Work out the finished part from the listing and answer in its coordinate system (mm). A direction names the side the tool comes from. Coordinates: 2 decimals unless noted, no trailing zeros. Order: outer loops, then holes, each group sorted by start corner. A loop starts at its lowest first (then second) coordinate and runs counter-clockwise, first axis right, second up. Notation, with made-up numbers: (-13.5, 35) -> (25.5, 35) arc R32 cw to (25.5, 71) -> close; hole circle Ø6 at (84.5, -32.75). An arc over 180 degrees is marked (long way). Answer as CSV lines item,"result". Start each with the question number.
Item 1: Section C-C (y = 26) is taken. Write down the section's boundary in (x, z), then the cut area to 3 significant figures.
Item 2: Straight lines are drawn through the part: L1, parallel to Y at x = 417.5, z = -29.5; L2, parallel to Z at x = -344, y = 48. For each, find the intervals that lie inside material, in ascending order.
Item 3: Each of these flat-tipped pins is pushed along its axis until it touches: pin 1 Ø3 at (x, y) = (123, 39.5) entering from -Z; pin 2 Ø1 at (x, z) = (-215.5, -22.5) entering from +Y. Where does it stop, or does it pass through?
Item 4: Section A-A (x = 196) is taken. Write down the section's boundary in (y, z).
Item 5: Section B-B (z = -20) is taken. Write down the section's boundary in (x, y), then the cut area to 3 significant figures.
Item 6: Which of the six approach directions +Z, -Z, +X, -X, +Y, -Y give full straight-line access (tool end or side, diameter ignored) to faces 1 (the face through (8, 32, 0)), 2 (the face through (8, 32, -3))?
```python
from build123d import *

# Parameters (mm, degrees)
BOSS_EXTRUDE1_DEPTH = 550
FILLET1_R           = 5
FILLET2_R           = 1


with BuildPart() as part:
    # Sketch1 → Boss-Extrude1 (new, symmetric)
    with BuildSketch(Plane(origin=(0, 0, 0), x_dir=(0, 0, -1), z_dir=(1, 0, 0))):
        Polygon((0, 0), (0, 60), (3, 60), (3, 3), (60, 3), (60, 0), align=None)
    extrude(amount=BOSS_EXTRUDE1_DEPTH, both=True)

    # Fillet1
    fillet1_edges = [part.edges().sort_by_distance(p)[0] for p in [
        (0, 0, 0),
    ]]
    fillet(fillet1_edges, radius=FILLET1_R)

    # Fillet2
    fillet2_edges = [part.edges().sort_by_distance(p)[0] for p in [
        (0, 3, -3),
    ]]
    fillet(fillet2_edges, radius=FILLET2_R)


solid = part.part
```
Checked values:
1,outline,"(-550, -3) -> (550, -3) -> (550, 0) -> (-550, 0) -> close"
1,area,"3,300 mm^2"
2,L1,"y = 0 to 3"
2,L2,"z = -3 to 0"
3,pin 1,"stops at z = -3"
3,pin 2,"stops at y = 3"
4,outline,"(0, -60) -> (3, -60) -> (3, -4) arc R1 cw to (4, -3) -> (60, -3) -> (60, 0) -> (5, 0) arc R5 ccw to (0, -5) -> close"
5,outline,"(-550, 0) -> (550, 0) -> (550, 3) -> (-550, 3) -> close"
5,area,"3,300 mm^2"
6,face 1,"+Z, +X, -X, +Y, -Y"
6,face 2,"-Z, +X, -X, +Y"
